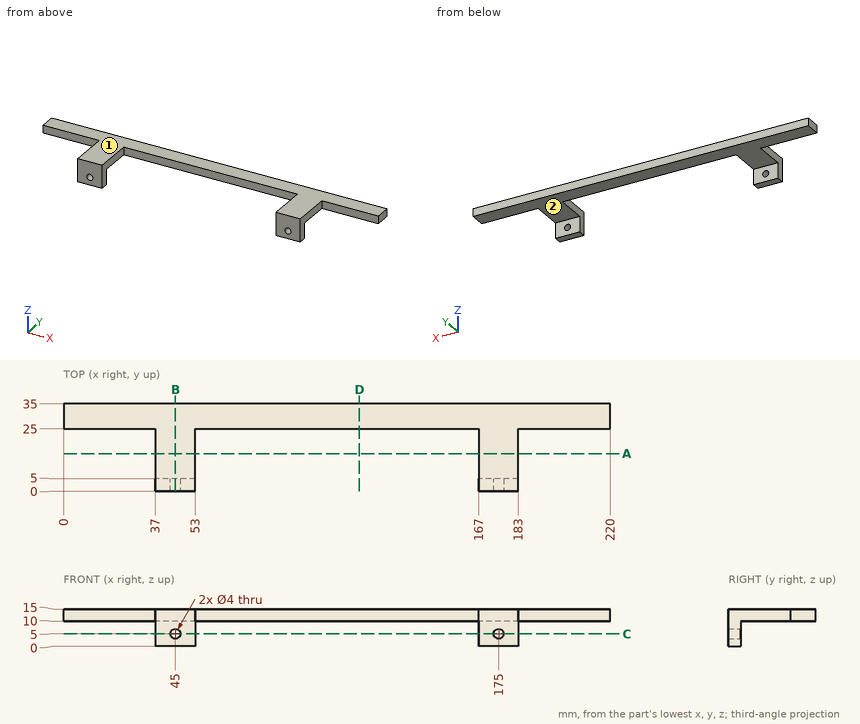
Design review of the part shown in the three views and the two pictorial views. Dimensions are in mm from the part's minimum x, y and z. A direction names the side the tool comes from. Coordinates: 2 decimals unless noted, no trailing zeros. Write each loop counter-clockwise with the first axis right and the second up, starting at its lowest first coordinate (ties: lowest second). Pieces come first, ordered by that corner, then holes.
1) We need section A-A on y = 15. State the section outline as (x, z) points, then the cut area to 3 significant figures.
2) We need section D-D on x = 119. State the section outline as (y, z) points, then the cut area to 3 significant figures.
3) Clearance check with flat-ended pins moving along their axes: pin 1 Ø7.5 at (y, z) = (17, 6.5) entering from -X; pin 2 Ø7.5 at (y, z) = (15, 9) entering from +X; pin 3 Ø5 at (x, z) = (175, 5) entering from -Y; pin 4 Ø4 at (x, z) = (111.5, 13.5) entering from -Y. State where each tip first meets the part, or that it passes through.
4) To check wall thickness, follow probe 1 along Z at (x, y) = (175, 3.6); probe 2 along Z at (x, y) = (58, 31); probe 3 along X at (y, z) = (3, 13). State the ranges of each line that lie inside material, in increasing order.
5) We need section B-B on x = 45. State the section outline as (y, z) points, then the cut area to 3 significant figures.
6) Machinability: for the marked faces 1 and 2, which of the approach directions +Z, -Z, +X, -X, +Y, -Y give a long, thin tool a straight path to every point of the face, cutting with its end or side? Answer none if there is none.
7) We need section C-C on z = 5. State the section outline as (x, y) points.
Answer list:
1. outline: (37, 10) - (53, 10) - (53, 15) - (37, 15) - close; (167, 10) - (183, 10) - (183, 15) - (167, 15) - close
1. area: 160 mm2
2. outline: (25, 10) - (35, 10) - (35, 15) - (25, 15) - close
2. area: 50.0 mm2
3. pin 1: stops at x = 37
3. pin 2: stops at x = 183
3. pin 3: stops at y = 0
3. pin 4: stops at y = 25
4. probe 1: z = 0 to 3, 7 to 15
4. probe 2: z = 10 to 15
4. probe 3: x = 37 to 53, 167 to 183
5. outline: (0, 0) - (5, 0) - (5, 3) - (0, 3) - close; (0, 7) - (5, 7) - (5, 10) - (35, 10) - (35, 15) - (0, 15) - close
5. area: 205 mm2
6. face 1: +Z, +X, -X, +Y, -Y
6. face 2: -Z, +X, -X, +Y
7. outline: (37, 0) - (43, 0) - (43, 5) - (37, 5) - close; (47, 0) - (53, 0) - (53, 5) - (47, 5) - close; (167, 0) - (173, 0) - (173, 5) - (167, 5) - close; (177, 0) - (183, 0) - (183, 5) - (177, 5) - close
